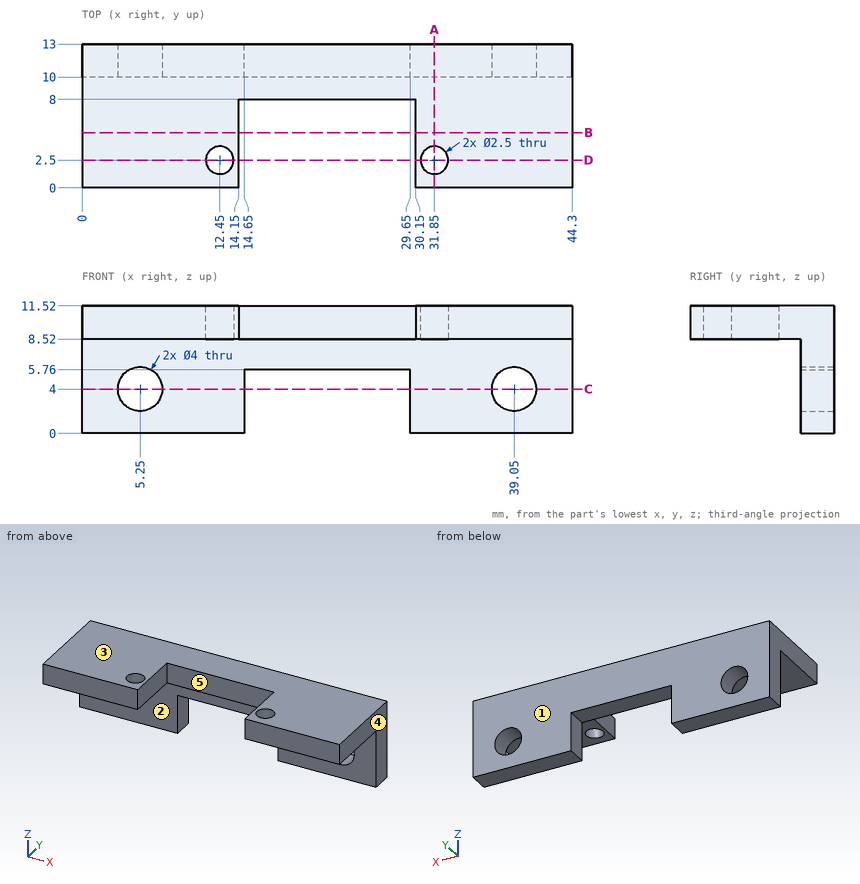
Design review of the part shown in the three views and the two pictorial views. Dimensions are in mm from the part's minimum x, y and z. A direction names the side the tool comes from. Coordinates: 2 decimals unless noted, no trailing zeros. Order: outer loops, then holes, each group sorted by start corner. A loop starts at its lowest first (then second) coordinate and runs counter-clockwise, first axis right, second up.
1) Take a section at B-B, the plane y = 5. Give the boundary of the cut face in (x, z), and give its area (3 significant figures).
2) Clearance check with flat-ended pins moving along their axes: pin 1 (1.5 mm diameter, centred on y = 8, z = 10, fed in from -X); pin 2 (6 mm diameter, centred on x = 31, z = 2, fed in from -Y); pin 3 (1 mm diameter, centred on x = 33.5, y = 2.5, fed in from -Z); pin 4 (1.5 mm diameter, centred on x = 20, z = 9.5, fed in from -Y). State where each tip first meets the part, or that it passes through.
3) Mouldability with a two-part tool opening along X and no side actions: class the marked faces 3, 4 and 5 as +X half, -X half, draft (parallel to the pull), parting line (faces both ways), or undercut.
4) Take a section at A-A, the plane x = 31.85. Give the boundary of the cut face in (y, z).
5) Take a section at C-C, the plane z = 4. Give the boundary of the cut face in (x, y), and give its area (3 significant figures).
6) Wall thickness on line 1 along X through (y, z) = (10.8, 4); line 2 along X through (y, z) = (12.5, 1.75); line 3 along Y through (x, z) = (31.85, 9.6): over which ranges is each line inside the solid? List them lowest first.
7) Take a section at D-D, the plane y = 2.5. Give the boundary of the cut face in (x, z), and give its area (3 significant figures).
8) For the marked faces 1 and 2, list the 3-axis set-ups (+Z, -Z, +X, -X, +Y, -Y) from which the entire face can be reached by the end or side of a thin tool; tool diameter is ignored.
Returned:
1. outline: (0, 8.52) - (14.15, 8.52) - (14.15, 11.52) - (0, 11.52) - close; (30.15, 8.52) - (44.3, 8.52) - (44.3, 11.52) - (30.15, 11.52) - close
1. area: 84.9 mm2
2. pin 1: stops at x = 0
2. pin 2: stops at y = 10
2. pin 3: stops at z = 8.52
2. pin 4: stops at y = 8
3. face 3: draft
3. face 4: +X half
3. face 5: undercut
4. outline: (0, 8.52) - (1.25, 8.52) - (1.25, 11.52) - (0, 11.52) - close; (3.75, 8.52) - (10, 8.52) - (10, 0) - (13, 0) - (13, 11.52) - (3.75, 11.52) - close
5. outline: (0, 10) - (3.25, 10) - (3.25, 13) - (0, 13) - close; (7.25, 10) - (14.65, 10) - (14.65, 13) - (7.25, 13) - close; (29.65, 10) - (37.05, 10) - (37.05, 13) - (29.65, 13) - close; (41.05, 10) - (44.3, 10) - (44.3, 13) - (41.05, 13) - close
5. area: 63.9 mm2
6. line 1: x = 0 to 3.25, 7.25 to 14.65, 29.65 to 37.05, 41.05 to 44.3
6. line 2: x = 0 to 14.65, 29.65 to 44.3
6. line 3: y = 0 to 1.25, 3.75 to 13
7. outline: (0, 8.52) - (11.2, 8.52) - (11.2, 11.52) - (0, 11.52) - close; (13.7, 8.52) - (14.15, 8.52) - (14.15, 11.52) - (13.7, 11.52) - close; (30.15, 8.52) - (30.6, 8.52) - (30.6, 11.52) - (30.15, 11.52) - close; (33.1, 8.52) - (44.3, 8.52) - (44.3, 11.52) - (33.1, 11.52) - close
7. area: 69.9 mm2
8. face 1: +Z, -Z, +X, -X, +Y
8. face 2: -Z, +X, -X, -Y
